Autodesk Inventor part; units mm, degrees
ref_plane "YZ Plane" through (0, 0, 0) normal (1, 0, 0) x (0, 1, 0)
ref_plane "XZ Plane" through (0, 0, 0) normal (0, 1, 0) x (-1, 0, 0)
ref_plane "XY Plane" through (0, 0, 0) normal (0, 0, 1) x (1, 0, 0)
sketch "Esboço1" plane through (0, 0, 0) normal (0, 0, 1) x (1, 0, 0)
  line L0 (-50.5, 39) -> (50.5, 39)
  line L1 (50.5, 39) -> (50.5, -39)
  line L2 (50.5, -39) -> (-50.5, -39)
  line L3 (-50.5, -39) -> (-50.5, 39)
  point P0 (0, 0)
  dimension "d2" = 101
  dimension "d3" = 78
  dimension "d4" = 101
  dimension "d5" = 50.5
  dimension "d6" = 39
extrude "Extrusão1" add sketch "Esboço1" against normal blind 2
sketch "Esboço2" plane through (0, 0, 0) normal (0, 0, 1) x (1, 0, 0)
  line L0 (50.5, -39) -> (-50.5, -39)
  line L1 (42.5, 39) -> (42.5, -39) construction
  line L2 (-50.5, -39) -> (-50.5, 39)
  line L3 (50.5, 39) -> (50.5, -39)
  line L4 (-42.5, 39) -> (-42.5, -39) construction
  line L5 (-50.5, 39) -> (50.5, 39)
  line L6 (-50.5, 19.5) -> (50.5, 19.5) construction
  line L7 (-50.5, -19.5) -> (50.5, -19.5) construction
  line L8 (-50.5, 39) -> (50.5, 39)
  line L9 (-46.5, 39) -> (-46.5, -39) construction
  line L10 (50.5, -39) -> (-50.5, -39)
  line L11 (46.5, 39) -> (46.5, -39) construction
  point P0 (0, 0)
  point P1 (-46.5, 19.5)
  point P2 (-46.5, -19.5)
  point P3 (46.5, -19.5)
  point P4 (46.5, 19.5)
  dimension "d32" = 8
  dimension "d33" = 8
  dimension "d34" = 4
  dimension "d35" = 4
  dimension "d36" = 19.5
  dimension "d37" = 58.5
  dimension "d38" = 78
  dimension "d39" = 78
hole "Furo2" at (-46.5, 19.5, 0) at (-46.5, -19.5, 0) at (46.5, -19.5, 0) at (46.5, 19.5, 0) direction (0, 0, -1) diameter 3 end through all counterbore diameter 6.5 counterbore depth 1.5
sketch "Esboço3" plane through (0, 0, 0) normal (0, 0, 1) x (1, 0, 0)
  line L0 (-22.0376, -18.7161) -> (-38.0376, -18.7161)
  line L1 (-38.0376, -18.7161) -> (-38.0376, -31.7161)
  line L2 (-22.0376, -31.7161) -> (-22.0376, -18.7161)
  line L3 (-38.0376, -31.7161) -> (-22.0376, -31.7161)
  line L4 (-39.6791, -31.6586) -> (39.7959, -31.6586)
  line L5 (-18.3542, -30.6586) -> (-17.2542, -30.6586)
  line L6 (-18.8542, -30.6586) -> (-18.3542, -30.6586)
  line L7 (-17.2542, -30.6586) -> (-16.7542, -30.6586)
  line L8 (-16.5542, -30.6586) -> (-16.7542, -30.6586)
  line L9 (-16.5542, -30.6586) -> (-16.5542, -30.6586)
  line L10 (-16.5542, -31.6586) -> (-16.5542, -30.6586)
  line L11 (-16.6542, -31.6586) -> (-16.5542, -31.6586)
  line L12 (-16.6542, -31.6586) -> (-17.0042, -31.6586)
  line L13 (-17.1042, -31.6586) -> (-17.0042, -31.6586)
  line L14 (-17.1042, -31.6586) -> (-17.6542, -31.6586)
  line L15 (-17.9542, -31.6586) -> (-17.6542, -31.6586)
  line L16 (-17.9542, -31.6586) -> (-18.9542, -31.6586)
  line L17 (-19.0542, -31.6586) -> (-18.7042, -31.6586)
  line L18 (-19.0542, -30.6586) -> (-19.0542, -31.6586)
  line L19 (-9.5679, -25.4931) -> (-14.5971, -25.4931)
  line L20 (12.8419, -28.4101) -> (10.7613, -25.4356)
  line L21 (10.7613, -31.6586) -> (10.7613, -25.4356)
  line L22 (12.8419, -29.4261) -> (12.8419, -28.4101)
  line L23 (-14.5971, -31.7161) -> (-14.5971, -25.4931)
  line L24 (-9.5679, -31.7161) -> (-9.5679, -25.4931)
  line L25 (-21.5376, -32.2161) -> (-38.5376, -32.2161)
  line L26 (-38.5376, -32.2161) -> (-38.5376, -18.2161)
  line L27 (-38.5376, -18.2161) -> (-21.5376, -18.2161)
  line L28 (-21.5376, -18.2161) -> (-21.5376, -32.2161)
  circle A0 centre (-17.8042, -31.1586) radius 1.5
  line L29 (-9.5679, -25.4356) -> (10.7613, -25.4356) construction
  line L30 (-5.4326, -25.4356) -> (6.5674, -25.4356)
  line L31 (-5.4326, -25.4356) -> (-5.4326, -17.4356)
  line L32 (-5.4326, -17.4356) -> (6.5674, -17.4356)
  line L33 (6.5674, -17.4356) -> (6.5674, -25.4356)
  line L34 (10.7029, -25.4356) -> (15.7321, -25.4356)
  line L35 (15.7321, -31.6586) -> (15.7321, -25.4356)
  line L36 (10.7029, -31.6586) -> (10.7029, -25.4356)
  line L37 (-14.5971, -31.6586) -> (-9.5679, -31.6586)
  line L38 (-9.5679, -31.6586) -> (-9.5679, -25.4356)
  line L39 (-14.5971, -25.4356) -> (-9.5679, -25.4356)
  line L40 (-14.5971, -31.6586) -> (-14.5971, -25.4356)
  point P0 (0, 0)
  point P1 (39.7959, -31.6586)
  dimension "d49" = 17
  dimension "d50" = 14
  dimension "d51" = 17
  dimension "d52" = 3
  dimension "d61" = 8
  dimension "d70" = 0.5
  dimension "d71" = 0
  dimension "d72" = 0.5
  dimension "d74" = 12
  dimension "d75" = 16.105
  dimension "d76" = 4.1355
  dimension "d77" = 4.1353
extrude "Extrusão2" cut sketch "Esboço3" against normal blind 10 contours L2 L4 L1 L0 | L0 L1 L4 L26 L27 L28 L2 | L4 L28 L25 L26 L1 L3 L2 | L2 L3 L1 L4 | A0 L4 | L4 A0 | L31 L32 L33 L30
equation "\"d2\" = 2 * d5"
equation "\"d3\" = 2 * d6"
equation "\"d4\" = d2"
equation "\"d33\" = d32"
equation "\"d34\" = d35"
equation "\"d35\" = 0.5 * d32"
properties part number "Ra-Manager_Painel-Placas" material "Aço, carbono"
For this review, take the finished solid that the model builds, in its own axes (mm). A direction names the side the tool comes from. Coordinates: 2 decimals unless noted, no trailing zeros. Write each loop counter-clockwise with the first axis right and the second up, starting at its lowest first coordinate (ties: lowest second). Pieces come first, ordered by that corner, then holes. Notation, with made-up numbers: (47, 60.5) -> (94, 60.5) arc R19 cw to (94, 97.5) -> close; hole circle Ø11 at (-29.5, -21). An arc over 180 degrees is marked (long way). Write each question's results on one line, items separated by ' | '. Start each with the question number.
1) Consider section A-A (x = -29.5). Write out the cut boundary in (y, z).
2) Consider section C-C (x = 46.5). Write out the cut boundary in (y, z), plus the area to 4 significant figures.
3) Insertion check: pin 1 (2 mm diameter, centred on x = 45, y = -20, fed in from +Z). The pin has a flat end and moves straight along its axis. Give the tip position at first contact, or say it passes through.
4) Consider section D-D (y = 19.5). Write out the cut boundary in (x, z), plus the area to 4 significant figures.
5) Wall thickness on L1, parallel to X at y = -19.5, z = -0.45; L2, parallel to Y at x = 46.5, z = -1.8; L3, parallel to Y at x = 46.5, z = -0.8: over which ranges is each line inside the solid? List them lowest first. Write a range as [from, to].
6) For faces 4 (the face through (-1, 1, 0)), 5 (the face through (-38.538, -25, -1)), 6 (the face through (45, -20.2, -1.5)), list the 3-axis set-ups (+Z, -Z, +X, -X, +Y, -Y) from which the entire face can be reached by the end or side of a thin tool; tool diameter is ignored.
7) Consider section B-B (y = -19.5). Write out the cut boundary in (x, z).
8) The part is to be moulded in two halves that separate along X. For faces 1 (the face through (-50.5, -1, -1)), 2 (the face through (-5.433, -21, -1)), 3 (the face through (-1, 39, -1)), say which applies: +X half, -X half, draft (parallel to the pull), parting line (faces both ways), or undercut.
Geometry says:
1) outline: (-39, -2) -> (-32.22, -2) -> (-32.22, 0) -> (-39, 0) -> close; (-18.22, -2) -> (39, -2) -> (39, 0) -> (-18.22, 0) -> close
2) outline: (-39, -2) -> (-21, -2) -> (-21, -1.5) -> (-22.75, -1.5) -> (-22.75, 0) -> (-39, 0) -> close; (-18, -2) -> (18, -2) -> (18, -1.5) -> (16.25, -1.5) -> (16.25, 0) -> (-16.25, 0) -> (-16.25, -1.5) -> (-18, -1.5) -> close; (21, -2) -> (39, -2) -> (39, 0) -> (22.75, 0) -> (22.75, -1.5) -> (21, -1.5) -> close | area: 133.5 mm^2
3) pin 1: z = -1.5
4) outline: (-50.5, -2) -> (-48, -2) -> (-48, -1.5) -> (-49.75, -1.5) -> (-49.75, 0) -> (-50.5, 0) -> close; (-45, -2) -> (45, -2) -> (45, -1.5) -> (43.25, -1.5) -> (43.25, 0) -> (-43.25, 0) -> (-43.25, -1.5) -> (-45, -1.5) -> close; (48, -2) -> (50.5, -2) -> (50.5, 0) -> (49.75, 0) -> (49.75, -1.5) -> (48, -1.5) -> close | area: 179.5 mm^2
5) L1: [-50.5, -49.75], [-43.25, -38.54], [-21.54, -5.43], [6.57, 43.25], [49.75, 50.5] | L2: [-39, -21], [-18, 18], [21, 39] | L3: [-39, -22.75], [-16.25, 16.25], [22.75, 39]
6) face 4: +Z, +X, -X, +Y, -Y | face 5: +Z, -Z | face 6: +Z
7) outline: (-50.5, -2) -> (-48, -2) -> (-48, -1.5) -> (-49.75, -1.5) -> (-49.75, 0) -> (-50.5, 0) -> close; (-45, -2) -> (-38.54, -2) -> (-38.54, 0) -> (-43.25, 0) -> (-43.25, -1.5) -> (-45, -1.5) -> close; (-21.54, -2) -> (-5.43, -2) -> (-5.43, 0) -> (-21.54, 0) -> close; (6.57, -2) -> (45, -2) -> (45, -1.5) -> (43.25, -1.5) -> (43.25, 0) -> (6.57, 0) -> close; (48, -2) -> (50.5, -2) -> (50.5, 0) -> (49.75, 0) -> (49.75, -1.5) -> (48, -1.5) -> close
8) face 1: -X half | face 2: undercut | face 3: draft
